Autodesk Fusion 360 part; units mm, degrees
sketch "Sketch1" plane through (0, 0, 0) normal (0, 0, 1) x (1, 0, 0)
  circle A0 centre (0, 0) radius 3.125
  circle A1 centre (0, 0) radius 19
  circle A2 centre (0, 0) radius 7.5
  circle A3 centre (0, 0) radius 15
  line L0 (-2, -6) -> (2, -6)
  line L1 (2, -6) -> (2, -16)
  line L2 (2, -16) -> (-2, -16)
  line L3 (-2, -16) -> (-2, -6)
  line L4 (4.1962, 4.7321) -> (12.8564, 9.7321)
  line L5 (14.8564, 6.2679) -> (6.1962, 1.2679)
  line L6 (-6.1962, 1.2679) -> (-14.8564, 6.2679)
  line L7 (-12.8564, 9.7321) -> (-4.1962, 4.7321)
  dimension "d1" = 6.25
  dimension "d2" = 38
  dimension "d3" = 15
  dimension "d5" = 360
extrude "Extrude1" add sketch "Sketch1" along normal blind 8 contours A1 | A2 L0 L1 L3 | A2 A3 L4 L5 | A2 A3 L1 L3 | A2 L0 L1 L3 | A3 L1 L2 L3 | A2 A3 L6 L7
Can you work these out from the model? Positions are in its coordinate system, mm. A direction names the side the tool comes from. Coordinates: 2 decimals unless noted, no trailing zeros. Write each loop counter-clockwise with the first axis right and the second up, starting at its lowest first coordinate (ties: lowest second). Pieces come first, ordered by that corner, then holes. Notation, with made-up numbers: (-2, 41) -> (15, 41) arc R23 cw to (15, 75) -> close; hole circle Ø2 at (1, -17.75). An arc over 180 degrees is marked (long way). Write each question's results on one line, items separated by ' | '. Start each with the question number.
Item 1: If we section it at A-A, the plane y = 0: Write out the boundary of the cut face in (x, z) (3 decimals), and give its area (3 significant figures).
Item 2: Please list where these lines run through material, in increasing order: probe 1 along Y at (x, z) = (0, 4.75) (3 decimals); probe 2 along X at (y, z) = (-10.5, 2.5); probe 3 along X at (y, z) = (-11, 4).
Item 3: If we section it at C-C, the plane z = 1.5: Write out the boundary of the cut face in (x, y) (3 decimals), and give its area (3 significant figures).
Item 4: Thinking about a two-plate mould opening in Y: for faces 1 (the cylindrical face through (8.767, 16.856, 3.944)), 2 (the flat face through (0, -4, 8)), 3 (the flat face through (10.614, 3.818, 3.944)), which applies, released by +Y, released by -Y, zero draft, split by the parting line, or undercut?
Item 5: If we section it at D-D, the plane y = -12.5: Write out the boundary of the cut face in (x, z).
Item 6: I'm going to push flat-ended pins straight in: P1, Ø1.5, axis at y = 5, z = 1, coming from the -X side; P2, Ø4, axis at y = -12, z = 3.5, coming from the +X side; P3, Ø3, axis at x = -3, y = 10, coming from the +Z side; P4, Ø1, axis at x = -6, z = 7, coming from the +Y side. Where does each tip first touch, or does it pass through?
Item 7: On a 3-axis mill with a long thin cutter (end or side, diameter ignored), from which of +Z, -Z, +X, -X, +Y, -Y can I reach the whole of each face in a straight line? I mean faces 4 (the flat face through (-10.521, 3.765, 3.944)), 5 (the flat face through (0, -4, 0)). Say none if no direction works.
Item 8: If we section it at B-B, the plane x = 0: Write out the boundary of the cut face in (y, z) (3 decimals), and give its area (3 significant figures).
Answer block:
1) outline: (-19, 0) -> (-15, 0) -> (-15, 8) -> (-19, 8) -> close; (-7.5, 0) -> (-3.125, 0) -> (-3.125, 8) -> (-7.5, 8) -> close; (3.125, 0) -> (7.5, 0) -> (7.5, 8) -> (3.125, 8) -> close; (15, 0) -> (19, 0) -> (19, 8) -> (15, 8) -> close | area: 134 mm²
2) probe 1: -19 to -3.125, 3.125 to 7.5, 15 to 19 | probe 2: -15.84 to -10.71, -2 to 2, 10.71 to 15.84 | probe 3: -15.49 to -10.2, -2 to 2, 10.2 to 15.49
3) outline: circle Ø38 at (0, 0); hole (-13.874, 5.701) arc R15 ccw to (-2, -14.866) -> (-2, -7.228) arc R7.5 cw to (-7.26, 1.882) -> close; hole (-11.874, 9.165) -> (-5.26, 5.346) arc R7.5 cw to (5.26, 5.346) -> (11.874, 9.165) arc R15 ccw to start; hole circle Ø6.25 at (0, 0); hole (2, -14.866) arc R15 ccw to (13.874, 5.701) -> (7.26, 1.882) arc R7.5 cw to (2, -7.228) -> close | area: 664 mm²
4) face 1: split by the parting line | face 2: zero draft | face 3: undercut
5) outline: (-14.31, 0) -> (-8.29, 0) -> (-8.29, 8) -> (-14.31, 8) -> close; (-2, 0) -> (2, 0) -> (2, 8) -> (-2, 8) -> close; (8.29, 0) -> (14.31, 0) -> (14.31, 8) -> (8.29, 8) -> close
6) P1: x = -18.52 | P2: x = 16.16 | P3: through | P4: y = 18.19
7) face 4: +Z, -Z | face 5: -Z, +X, -X, +Y, -Y
8) outline: (-19, 0) -> (-3.125, 0) -> (-3.125, 8) -> (-19, 8) -> close; (3.125, 0) -> (7.5, 0) -> (7.5, 8) -> (3.125, 8) -> close; (15, 0) -> (19, 0) -> (19, 8) -> (15, 8) -> close | area: 194 mm²
